```python
from build123d import *

# Parameters (mm, degrees)
IZIM1_R                     = 32
Y_KSEKLIK_EKSTR_ZYON1_DEPTH = 70
IZIM2_R                     = 40
Y_KSEKLIK_EKSTR_ZYON2_DEPTH = 10
IZIM3_R                     = 40
Y_KSEKLIK_EKSTR_ZYON3_DEPTH = 15
IZIM4_W                     = 32
IZIM4_H                     = 32
KES_EKSTR_ZYON1_DEPTH       = 91
IZIM5_W                     = 10
IZIM5_H                     = 45
Y_KSEKLIK_EKSTR_ZYON6_DEPTH = 52.5
IZIM11_R                    = 9
KES_EKSTR_ZYON2_DEPTH       = 144.472343967
KES_EKSTR_ZYON3_DEPTH       = 144.472344097


with BuildPart() as part:
    # Çizim1 → Yükseklik-Ekstrüzyon1 (new body)
    with BuildSketch(Plane(origin=(0, 0, 0), x_dir=(1, 0, 0), z_dir=(0, 1, 0))):
        with Locations(Location((0, 0, 0), (0, 0, 270))):
            Circle(IZIM1_R)
    extrude(amount=Y_KSEKLIK_EKSTR_ZYON1_DEPTH)

    # Çizim2 → Yükseklik-Ekstrüzyon2 (add)
    with BuildSketch(Plane(origin=(0, 10, 0), x_dir=(1, 0, 0), z_dir=(0, 1, 0))):
        with Locations(Location((0, 0, 0), (0, 0, 270))):
            Circle(IZIM2_R)
    extrude(amount=Y_KSEKLIK_EKSTR_ZYON2_DEPTH)

    # Çizim3 → Yükseklik-Ekstrüzyon3 (add)
    with BuildSketch(Plane(origin=(0, 55, 0), x_dir=(1, 0, 0), z_dir=(0, 1, 0))):
        with Locations(Location((0, 0, 0), (0, 0, 270))):
            Circle(IZIM3_R)
    extrude(amount=Y_KSEKLIK_EKSTR_ZYON3_DEPTH)

    # Çizim4 → Kes-Ekstrüzyon1 (cut, through all)
    with BuildSketch(Plane(origin=(0, 70, 0), x_dir=(1, 0, 0), z_dir=(0, 1, 0))):
        Rectangle(IZIM4_W, IZIM4_H)
    extrude(amount=-KES_EKSTR_ZYON1_DEPTH, mode=Mode.SUBTRACT)

    # Çizim5 → Yükseklik-Ekstrüzyon6 (add)
    with BuildSketch(Plane(origin=(0, 70, 0), x_dir=(1, 0, 0), z_dir=(0, 1, 0))):
        with Locations((-28.071891388, 0)):
            Rectangle(IZIM5_W, IZIM5_H)
        with BuildLine():
            ThreePointArc((-33.071891388, 22.5), (-40, 0), (-33.071891388, -22.5))
            Line((-33.071891388, -22.5), (-33.071891388, 22.5))
        make_face()
        with Locations((28.071891388, 0)):
            Rectangle(IZIM5_W, IZIM5_H)
        with BuildLine():
            Line((33.071891388, 22.5), (33.071891388, -22.5))
            ThreePointArc((33.071891388, -22.5), (38.228756555, -11.771243445), (40, 0))
            ThreePointArc((40, 0), (38.228756555, 11.771243445), (33.071891388, 22.5))
        make_face()
    extrude(amount=Y_KSEKLIK_EKSTR_ZYON6_DEPTH)

    # Çizim11 → Kes-Ekstrüzyon2 (cut, through all)
    with BuildSketch(Plane.ZY.offset(-23.071891388)):
        with Locations((0, 100)):
            Circle(IZIM11_R)
        with BuildLine():
            ThreePointArc((-22.5, 100), (-15.909902516, 115.909902637), (1.71e-07, 122.5))
            Line((1.71e-07, 122.5), (-22.5, 122.5))
            Line((-22.5, 122.5), (-22.5, 100))
        make_face()
        with BuildLine():
            ThreePointArc((1.71e-07, 122.5), (15.909902637, 115.909902516), (22.5, 100))
            Line((22.5, 100), (22.5, 122.5))
            Line((22.5, 122.5), (1.71e-07, 122.5))
        make_face()
    extrude(amount=-KES_EKSTR_ZYON2_DEPTH, mode=Mode.SUBTRACT)

    # Çizim12 → Kes-Ekstrüzyon3 (cut, through all)
    with BuildSketch(Plane(origin=(-23.071891388, 0, 0), x_dir=(0, 0, -1), z_dir=(1, 0, 0))):
        with BuildLine():
            ThreePointArc((-22.5, 100), (-15.90990258, 115.909902574), (-8e-09, 122.5))
            Line((-8e-09, 122.5), (-22.5, 122.5))
            Line((-22.5, 122.5), (-22.5, 100))
        make_face()
        with BuildLine():
            ThreePointArc((-9, 100), (0, 91), (9, 100))
            Line((9, 100), (-9, 100))
        make_face()
        with BuildLine():
            Line((-9, 100), (9, 100))
            ThreePointArc((9, 100), (0, 109), (-9, 100))
        make_face()
        with BuildLine():
            ThreePointArc((-8e-09, 122.5), (15.909902574, 115.90990258), (22.5, 100))
            Line((22.5, 100), (22.5, 122.5))
            Line((22.5, 122.5), (-8e-09, 122.5))
        make_face()
    extrude(amount=-KES_EKSTR_ZYON3_DEPTH, mode=Mode.SUBTRACT)


solid = part.part
```
Source: CAD feature listing. Evaluate the final solid. Frame: model axes, mm. A direction names the side the tool comes from. Round coordinates to 2 decimals unless told otherwise and drop trailing zeros. Loops run counter-clockwise (first coordinate to the right, second up) from the corner with the lowest first, then second, coordinate; pieces in that order, holes last. Notation, with made-up numbers: M 24,-21.5 L 42,-21.5 A13 ccw 42,-6.5 Z; hole C 33,0 d1. An arc over 180 degrees is marked long. Use a Markdown table: item, result. Add a question column.
1. Section query D-D on y = 60.5. Return the cut outline in (x, z), then the cut area to 3 significant figures.
2. Section query C-C on z = -26.5. Return the cut outline in (x, y), then the cut area to 3 significant figures.
3. Line query: line 1 (Y direction, x = 34, z = 0); line 2 (Z direction, x = 33, y = 100); line 3 (Y direction, x = 6.5, z = -31). Output: solid intervals per line, ascending.
4. Mould query, pull axis X, two halves, no side actions, for faces 1 (the cylindrical face through (-31.24, 4.93, -6.94)), 2 (the flat face through (0, 35, -16)), 3 (the cylindrical face through (31.417, 91.214, -1.951)), 4 (the flat face through (-23.072, 90, 0)). Classes: pulls with the +X half, pulls with the -X half, needs draft (parallel to the pull), parting line crosses it, or undercut.
5. Section query A-A on x = 0. Return the cut outline in (y, z).
6. Section query B-B on y = 38. Return the cut outline in (x, z), then the cut area to 3 significant figures.
7. Contact query for flat-ended pins moving along their axis: P1, Ø1.5, axis at x = -23, z = 14, coming from the +Y side; P2, Ø8, axis at y = 30, z = -6, coming from the +X side; P3, Ø1, axis at y = 20, z = 12, coming from the -X side. Output: stop coordinate, or through.
8. Reachability of faces 5 (the flat face through (-16, 35, 0)), 6 (the flat face through (-28, 85, 22.5)), 7 (the flat face through (23.072, 90, 0)) from +Z, -Z, +X, -X, +Y, -Y: full face, straight path, thin tool, end or side. Return the list, or none.
Reported:
| question | item | result |
|---|---|---|
| 1 | outline | C 0,0 d80; hole M -16,-16 L 16,-16 L 16,16 L -16,16 Z |
| 1 | area | 4,000 mm² |
| 2 | outline | M -29.96,10 L -17.94,10 L -17.94,0 L 17.94,0 L 17.94,10 L 29.96,10 L 29.96,20 L 17.94,20 L 17.94,55 L 29.96,55 L 29.96,70 L -29.96,70 L -29.96,55 L -17.94,55 L -17.94,20 L -29.96,20 Z |
| 2 | area | 3,110 mm² |
| 3 | line 1 | y = 10 to 20, 55 to 91, 109 to 122.5 |
| 3 | line 2 | z = -22.5 to -9, 9 to 22.5 |
| 3 | line 3 | y = 0 to 70 |
| 4 | face 1 | parting line crosses it |
| 4 | face 2 | undercut |
| 4 | face 3 | needs draft |
| 4 | face 4 | undercut |
| 5 | outline | M 0,-32 L 10,-32 L 10,-40 L 20,-40 L 20,-32 L 55,-32 L 55,-40 L 70,-40 L 70,-16 L 0,-16 Z; M 0,16 L 70,16 L 70,40 L 55,40 L 55,32 L 20,32 L 20,40 L 10,40 L 10,32 L 0,32 Z |
| 6 | outline | C 0,0 d64; hole M -16,-16 L 16,-16 L 16,16 L -16,16 Z |
| 6 | area | 2,190 mm² |
| 7 | P1 | stops at y = 118.18 |
| 7 | P2 | stops at x = 31.94 |
| 7 | P3 | stops at x = -38.31 |
| 8 | face 5 | +Y, -Y |
| 8 | face 6 | +Z, +X, -X, +Y |
| 8 | face 7 | +Z, -Z, +Y |
